```python
from build123d import *

# Parameters (mm, degrees)
BOSS_EXTRUDE1_DEPTH = 61
SKETCH2_R           = 3
CUT_EXTRUDE1_DEPTH  = 93.136108557
SKETCH3_R           = 4
CUT_EXTRUDE2_DEPTH  = 98.077610704
CUT_EXTRUDE3_START  = -16
SKETCH3_4_R         = 6.5
SKETCH3_4_R_2       = 4
CUT_EXTRUDE3_DEPTH  = 61
FILLET1_R           = 3


with BuildPart() as part:
    # Sketch1 → Boss-Extrude1 (new body)
    with BuildSketch(Plane(origin=(0, 0, 0), x_dir=(1, 0, 0), z_dir=(0, 1, 0))):
        with BuildLine():
            Line((40, 0), (0, 0))
            Line((0, 0), (-40, 0))
            Line((-40, 0), (-40, -20))
            Line((-40, -20), (-40, -41.75))
            Line((-40, -41.75), (-55, -41.75))
            Line((-55, -41.75), (-55, -51.75))
            Line((-55, -51.75), (-40, -51.75))
            Line((-40, -51.75), (-31.75, -51.75))
            ThreePointArc((-31.75, -51.75), (0, -20), (31.75, -51.75))
            Line((31.75, -51.75), (40, -51.75))
            Line((40, -51.75), (55, -51.75))
            Line((55, -51.75), (55, -41.75))
            Line((55, -41.75), (40, -41.75))
            Line((40, -41.75), (40, -20))
            Line((40, -20), (40, 0))
        make_face()
    extrude(amount=BOSS_EXTRUDE1_DEPTH)

    # Sketch2 → Cut-Extrude1 (cut, through all)
    with BuildSketch(Plane(origin=(0, 0, 41.75), x_dir=(-1, 0, 0), z_dir=(0, 0, -1))):
        with Locations((-47.5, 51)):
            Circle(SKETCH2_R)
        with Locations((-47.5, 10)):
            Circle(SKETCH2_R)
        with Locations(Location((47.5, 10, 0), (0, 0, 180))):
            Circle(SKETCH2_R)
        with Locations(Location((47.5, 51, 0), (0, 0, 180))):
            Circle(SKETCH2_R)
    extrude(amount=-CUT_EXTRUDE1_DEPTH, mode=Mode.SUBTRACT)

    # Sketch3 → Cut-Extrude2 (cut, through all)
    with BuildSketch(Plane(origin=(0, 0, 0), x_dir=(-1, 0, 0), z_dir=(0, 0, -1))):
        with Locations((-20, 47)):
            Circle(SKETCH3_R)
        with Locations((-20, 14)):
            Circle(SKETCH3_R)
        with Locations((20, 14)):
            Circle(SKETCH3_R)
        with Locations((20, 47)):
            Circle(SKETCH3_R)
    extrude(amount=-CUT_EXTRUDE2_DEPTH, mode=Mode.SUBTRACT)

    # Sketch3_4 → Cut-Extrude3 (cut)
    # profile 1 of 4: a face of its own
    with BuildSketch(Plane(origin=(0, 0, 0), x_dir=(-1, 0, 0), z_dir=(0, 0, -1)).offset(CUT_EXTRUDE3_START)):
        with Locations((-20, 47)):
            Circle(SKETCH3_4_R)
        with Locations((-20, 47)):
            Circle(SKETCH3_4_R_2, mode=Mode.SUBTRACT)
    # profile 2 of 4: a face of its own
    with BuildSketch(Plane(origin=(0, 0, 0), x_dir=(-1, 0, 0), z_dir=(0, 0, -1)).offset(CUT_EXTRUDE3_START)):
        with Locations((-20, 14)):
            Circle(SKETCH3_4_R)
        with Locations((-20, 14)):
            Circle(SKETCH3_4_R_2, mode=Mode.SUBTRACT)
    # profile 3 of 4: a face of its own
    with BuildSketch(Plane(origin=(0, 0, 0), x_dir=(-1, 0, 0), z_dir=(0, 0, -1)).offset(CUT_EXTRUDE3_START)):
        with Locations((20, 14)):
            Circle(SKETCH3_4_R)
        with Locations((20, 14)):
            Circle(SKETCH3_4_R_2, mode=Mode.SUBTRACT)
    # profile 4 of 4: a face of its own
    with BuildSketch(Plane(origin=(0, 0, 0), x_dir=(-1, 0, 0), z_dir=(0, 0, -1)).offset(CUT_EXTRUDE3_START)):
        with Locations((20, 47)):
            Circle(SKETCH3_4_R)
        with Locations((20, 47)):
            Circle(SKETCH3_4_R_2, mode=Mode.SUBTRACT)
    extrude(amount=-CUT_EXTRUDE3_DEPTH, mode=Mode.SUBTRACT)

    # Fillet1
    fillet1_edges = [part.edges().sort_by_distance(p)[0] for p in [
        (-40, 30.5, 41.75),
        (40, 30.5, 41.75),
    ]]
    fillet(fillet1_edges, radius=FILLET1_R)


solid = part.part
```
Verification items for the finished model (mm, model axes). A direction names the side the tool comes from. Coordinates: 2 decimals unless noted, no trailing zeros. Loops run counter-clockwise (first coordinate to the right, second up) from the corner with the lowest first, then second, coordinate; pieces in that order, holes last. Notation, with made-up numbers: (-15, 55.5) - (20, 55.5) arc R29 ccw to (20, 86.5) - close; hole circle Ø5 at (17.25, 73). An arc over 180 degrees is marked (long way). Return JSON: item names as keys, results as strings.
1. Section check C-C, the plane z = 9. Record the boundary of the cut face in (x, y), then the cut area to 3 significant figures.
Established:
{"outline": "(-40, 0) - (40, 0) - (40, 61) - (-40, 61) - close; hole circle Ø8 at (-20, 14); hole circle Ø8 at (-20, 47); hole circle Ø8 at (20, 14); hole circle Ø8 at (20, 47)", "area": "4,680 mm2"}
2. Section check D-D, the plane x = 0. Record the boundary of the cut face in (y, z), then the cut area to 3 significant figures.
Established:
{"outline": "(0, 0) - (61, 0) - (61, 20) - (0, 20) - close", "area": "1,220 mm2"}
3. Mould release check, pull along X, two halves, no side actions. Record for faces 1 (the flat face through (17, 50, 16)), 2 (the cylindrical face through (40.86, 30.93, 40.85)), 3 (the flat face through (49, 30, 41.75)): +X half, -X half, draft (parallel to the pull), parting line (faces both ways), or undercut.
Established:
{"face 1": "undercut", "face 2": "+X half", "face 3": "draft"}
4. Go/stop test with flat-tipped pins: pin 1 (6 mm diameter, centred on y = 16, z = 5.5, fed in from -X); pin 2 (5 mm diameter, centred on y = 36.5, z = 13.5, fed in from +X); pin 3 (6 mm diameter, centred on x = 47, y = 29, fed in from -Z). Record where each tip stops, or that it passes through.
Established:
{"pin 1": "stops at x = -40", "pin 2": "stops at x = 40", "pin 3": "stops at z = 41.75"}
5. Tool access check on faces 4 (the flat face through (17, 17, 16)), 5 (the flat face through (-49, 30, 41.75)), 6 (the cylindrical face through (23.2, 44.6, 7.9)). Record the directions out of +Z, -Z, +X, -X, +Y, -Y that give a thin tool (end or side, any length) a straight path to the whole face; none if there is none.
Established:
{"face 4": "+Z", "face 5": "-Z, -X, +Y, -Y", "face 6": "+Z, -Z"}
6. Section check A-A, the plane x = -47.5. Record the boundary of the cut face in (y, z).
Established:
{"outline": "(0, 41.75) - (7, 41.75) - (7, 51.75) - (0, 51.75) - close; (13, 41.75) - (48, 41.75) - (48, 51.75) - (13, 51.75) - close; (54, 41.75) - (61, 41.75) - (61, 51.75) - (54, 51.75) - close"}
7. Section check B-B, the plane z = 30. Record the boundary of the cut face in (x, y).
Established:
{"outline": "(-40, 0) - (-23.13, 0) - (-23.13, 8.3) arc R6.5 cw to (-23.13, 19.7) - (-23.13, 41.3) arc R6.5 cw to (-23.13, 52.7) - (-23.13, 61) - (-40, 61) - close; (23.13, 0) - (40, 0) - (40, 61) - (23.13, 61) - (23.13, 52.7) arc R6.5 cw to (23.13, 41.3) - (23.13, 19.7) arc R6.5 cw to (23.13, 8.3) - close"}
8. Thickness scan on L1, parallel to Y at x = 20, z = 26; L2, parallel to X at y = 47, z = 26.25; L3, parallel to Y at x = 20, z = 4. Record the ranges inside material, lowest first.
Established:
{"L1": "y = 0 to 7.5, 20.5 to 40.5, 53.5 to 61", "L2": "x = -40 to -26.5, 26.5 to 40", "L3": "y = 0 to 10, 18 to 43, 51 to 61"}
